Work out the finished part from the listing and answer in its coordinate system (mm). Face numbers are marked on the shaded views. A direction names the side the tool comes from. Give positions to 0.01 mm unless a question says otherwise; leave off trailing zeros. Write each loop counter-clockwise with the first axis right and the second up, starting at its lowest first coordinate (ties: lowest second). Pieces come first, ordered by that corner, then holes. Notation, with made-up numbers: (37, 44.25) - (89, 44.25) arc R14 ccw to (89, 60.25) - close; hole circle Ø1 at (2.25, 2.5). An arc over 180 degrees is marked (long way). Write item = value, one per line.
from build123d import *

# Parameters (mm, degrees)
SKETCH1_W            = 75
SKETCH1_H            = 40
BOSS_EXTRUDE1_DEPTH  = 2
SKETCH2_W            = 75
SKETCH2_H            = 40
SKETCH2_W_2          = 71
SKETCH2_H_2          = 17
BOSS_EXTRUDE2_DEPTH  = 17
CUT_EXTRUDE2_DEPTH   = 17
CUT_EXTRUDE3_REACH   = 82.169
CUT_EXTRUDE4_REACH   = 88.683
SKETCH5_R            = 1.6
MIRROR2_COPY_1_DEPTH = 17


with BuildPart() as part:
    # Sketch1 → Boss-Extrude1 (new body)
    with BuildSketch(Plane(origin=(0, 0, 0), x_dir=(1, 0, 0), z_dir=(0, 1, 0))):
        with Locations((37.5, 20)):
            Rectangle(SKETCH1_W, SKETCH1_H)
    boss_extrude1 = extrude(amount=BOSS_EXTRUDE1_DEPTH)

    # Sketch2 → Boss-Extrude2 (add)
    with BuildSketch(Plane(origin=(0, 2, 0), x_dir=(1, 0, 0), z_dir=(0, 1, 0))):
        with Locations((37.5, 20)):
            Rectangle(SKETCH2_W, SKETCH2_H)
        with Locations((37.5, 29.5)):
            Rectangle(SKETCH2_W_2, SKETCH2_H_2, mode=Mode.SUBTRACT)
        with Locations((37.5, 10.5)):
            Rectangle(SKETCH2_W_2, SKETCH2_H_2, mode=Mode.SUBTRACT)
    boss_extrude2 = extrude(amount=BOSS_EXTRUDE2_DEPTH)

    # Sketch3 → Cut-Extrude2 (cut)
    with BuildSketch(Plane.XY):
        with BuildLine():
            Line((2, 17.5), (2, 19))
            Line((2, 19), (73, 19))
            Line((73, 19), (73, 17.5))
            ThreePointArc((73, 17.5), (70.5, 15), (68, 17.5))
            Line((68, 17.5), (49, 17.5))
            Line((49, 17.5), (46, 15))
            Line((46, 15), (29, 15))
            Line((29, 15), (26, 17.5))
            Line((26, 17.5), (7, 17.5))
            ThreePointArc((7, 17.5), (4.5, 15), (2, 17.5))
        make_face()
    cut_extrude2 = extrude(amount=-CUT_EXTRUDE2_DEPTH, mode=Mode.SUBTRACT)

    # Mirror1: Cut-Extrude2 across plane
    add(cut_extrude2.mirror(Plane.XY.offset(-20)), mode=Mode.SUBTRACT)

    # Sketch4 → Cut-Extrude3 (cut, up to next)
    with BuildSketch(Plane.XY.offset(-19), mode=Mode.PRIVATE) as cut_extrude3_sk1:
        Polygon((2, 18), (7.035918341, 18), (10.035918341, 15), (64.964081659, 15), (67.964081659, 18), (73, 18), (73, 19), (2, 19), align=None)
    cut_extrude3_tool1 = extrude(cut_extrude3_sk1.sketch, amount=-CUT_EXTRUDE3_REACH, mode=Mode.PRIVATE) & part.part
    cut_extrude3 = cut_extrude3_tool1.solids().sort_by_distance((37.5, 17.098486, -19))[0]
    add(cut_extrude3, mode=Mode.SUBTRACT)

    # Sketch5 → Cut-Extrude4 (cut, up to next)
    with BuildSketch(Plane(origin=(0, 2, 0), x_dir=(1, 0, 0), z_dir=(0, 1, 0)), mode=Mode.PRIVATE) as cut_extrude4_sk1:
        with Locations(Location((37.5, 29.5, 0), (0, 0, 270))):
            Circle(SKETCH5_R)
    cut_extrude4_tool1 = extrude(cut_extrude4_sk1.sketch, amount=-CUT_EXTRUDE4_REACH, mode=Mode.PRIVATE) & part.part
    # Sketch5 → Cut-Extrude4 (cut, up to next)
    with BuildSketch(Plane(origin=(0, 2, 0), x_dir=(1, 0, 0), z_dir=(0, 1, 0)), mode=Mode.PRIVATE) as cut_extrude4_sk2:
        with Locations(Location((37.5, 10.5, 0), (0, 0, 270))):
            Circle(SKETCH5_R)
    cut_extrude4_tool2 = extrude(cut_extrude4_sk2.sketch, amount=-CUT_EXTRUDE4_REACH, mode=Mode.PRIVATE) & part.part
    cut_extrude4_1 = cut_extrude4_tool1.solids().sort_by_distance((37.5, 2, -29.5))[0]
    add(cut_extrude4_1, mode=Mode.SUBTRACT)
    cut_extrude4_2 = cut_extrude4_tool2.solids().sort_by_distance((37.5, 2, -10.5))[0]
    add(cut_extrude4_2, mode=Mode.SUBTRACT)
    cut_extrude4 = cut_extrude4_1 + cut_extrude4_2  # Cut-Extrude4 as one shape, for the pattern or mirror that repeats it

    # Mirror2: Boss-Extrude1, Boss-Extrude2, Cut-Extrude2, Cut-Extrude3, Cut-Extrude4 across plane
    add(boss_extrude1.mirror(Plane.XY.offset(-1)))
    add(boss_extrude2.mirror(Plane.XY.offset(-1)))
    add(cut_extrude2.mirror(Plane.XY.offset(-1)), mode=Mode.SUBTRACT)
    add(cut_extrude3.mirror(Plane.XY.offset(-1)), mode=Mode.SUBTRACT)
    add(cut_extrude4.mirror(Plane.XY.offset(-1)), mode=Mode.SUBTRACT)

    # Mirror2 copy 1 sketch → Mirror2 copy 1 (cut)
    with BuildSketch(Plane.XY.offset(38)):
        with BuildLine():
            Line((2, 17.5), (2, 19))
            Line((2, 19), (73, 19))
            Line((73, 19), (73, 17.5))
            ThreePointArc((73, 17.5), (70.5, 15), (68, 17.5))
            Line((68, 17.5), (49, 17.5))
            Line((49, 17.5), (46, 15))
            Line((46, 15), (29, 15))
            Line((29, 15), (26, 17.5))
            Line((26, 17.5), (7, 17.5))
            ThreePointArc((7, 17.5), (4.5, 15), (2, 17.5))
        make_face()
    extrude(amount=-MIRROR2_COPY_1_DEPTH, mode=Mode.SUBTRACT)


solid = part.part
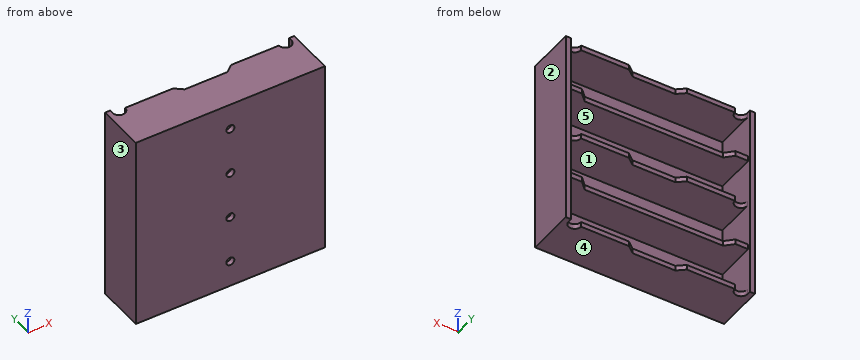
1. A tool of negligible diameter and unlimited length cuts with its end or side. For the marked faces 4 and 5, from which of +Z, -Z, +X, -X, +Y, -Y can it reach the whole face along a straight path? Write none if from no direction.
Solution:
face_4 = -Z, +X, -X, +Y, -Y
face_5 = +Y
2. Find section B-B, the plane x = 58. Give the vertices of the cut face in (y, z).
Solution:
outline = (0, -40) - (17.5, -40) - (17.5, -38) - (2, -38) - (2, -21) - (15, -21) - (15, -19) - (2, -19) - (2, -2) - (17.5, -2) - (17.5, 0) - (2, 0) - (2, 17) - (15, 17) - (15, 19) - (2, 19) - (2, 36) - (17.5, 36) - (17.5, 38) - (0, 38) - close
3. Find section C-C, the plane y = 8. Give the vertices of the cut face in (x, z).
Solution:
outline = (0, -40) - (75, -40) - (75, 38) - (0, 38) - close; hole (2, -38) - (73, -38) - (73, -21) - (2, -21) - close; hole (2, -19) - (73, -19) - (73, -2) - (2, -2) - close; hole (2, 0) - (73, 0) - (73, 17) - (2, 17) - close; hole (2, 19) - (73, 19) - (73, 36) - (2, 36) - close
4. Find section D-D, the plane x = 70.5. Give the vertices of the cut face in (y, z), then the cut area to 3 significant figures.
Solution:
outline = (0, -40) - (15, -40) - (15, -38) - (2, -38) - (2, -21) - (18, -21) - (18, -19) - (2, -19) - (2, -2) - (15, -2) - (15, 0) - (2, 0) - (2, 17) - (18, 17) - (18, 19) - (2, 19) - (2, 36) - (15, 36) - (15, 38) - (0, 38) - close
area = 298 mm^2
5. Straight lines are drawn through the part: line 1 (Z direction, x = 11, y = 12.75); line 2 (Z direction, x = 9.5, y = 16.75); line 3 (X direction, y = 17.75, z = -29.5). For each, find the intervals that lie inside material, in ascending order.
Solution:
line_1 = -40 to -38, -21 to -19, -2 to 0, 17 to 19, 36 to 38
line_2 = -40 to -38, -2 to 0, 36 to 38
line_3 = 0 to 2, 73 to 75
6. For a pull along X with two mould halves and no side action, classify the marked faces 1, 2 and 3 as pulls with the +X half, pulls with the -X half, needs draft (parallel to the pull), parting line crosses it, or undercut.
Solution:
face_1 = undercut
face_2 = pulls with the +X half
face_3 = pulls with the -X half
7. Given pin 1 (4 mm diameter, centred on x = 59, z = -7.5, fed in from +Y); pin 2 (0.6 mm diameter, centred on x = 55.5, z = -39.5, fed in from +Y); pin 3 (0.6 mm diameter, centred on x = 69.5, z = 18, fed in from +Y), each flat-ended and moving along its own axis, determine where each tip first touches the part or whether it passes through.
Solution:
pin_1 = 2
pin_2 = 17.5
pin_3 = 18
8. Find section A-A, the plane z = 27.5. Give the vertices of the cut face in (x, y).
Solution:
outline = (0, 0) - (35.9, 0) - (35.9, 2) - (2, 2) - (2, 19) - (0, 19) - close; (39.1, 0) - (75, 0) - (75, 19) - (73, 19) - (73, 2) - (39.1, 2) - close
